Build history of the part. All positions in model axes, mm. A direction names the side the tool comes from. Round coordinates to 2 decimals unless told otherwise and drop trailing zeros. Loops run counter-clockwise (first coordinate to the right, second up) from the corner with the lowest first, then second, coordinate; pieces in that order, holes last.
from build123d import *

# Parameters (mm, degrees)
F0_W     = 6
F0_H     = 8.2
F0_W_2   = 17.4
F0_H_2   = 3
F1_DEPTH = 7.5


with BuildPart() as f1:
    # F0 (on Front) → F1 (new body, symmetric)
    with BuildSketch(Plane.XZ):
        Polygon((-49.911916, 14.810329), (-49.911916, 9.810329), (46.088084, 9.810329), (50.088084, 9.810329), (50.088084, 14.810329), (19.588084, 14.810329), (13.588084, 14.810329), (-43.911916, 14.810329), align=None)
        with Locations((16.588084, 18.910329)):
            Rectangle(F0_W, F0_H)
        with Locations((-46.911916, 18.910329)):
            Rectangle(F0_W, F0_H)
        Polygon((50.088084, 9.810329), (46.088084, 9.810329), (46.088084, -5.289671), (46.088084, -8.289671), (46.088084, -11.489671), (46.088084, -14.489671), (50.088084, -14.489671), align=None)
        with Locations((37.388084, -6.789671)):
            Rectangle(F0_W_2, F0_H_2)
        with Locations((37.388084, -12.989671)):
            Rectangle(F0_W_2, F0_H_2)
    extrude(amount=F1_DEPTH, both=True)


solid = f1.part
(1) Probe line 1 (Z direction, x = 32.5, y = 4); line 2 (X direction, y = -5.25, z = 20); line 3 (Z direction, x = 16, y = -7). List the from-to ranges inside material, lowest first.
Responses:
line 1: z = -14.49 to -11.49, -8.29 to -5.29, 9.81 to 14.81
line 2: x = -49.91 to -43.91, 13.59 to 19.59
line 3: z = 9.81 to 23.01
(2) Pull direction X, two halves, no side cores. Call faces 1 (the face through (28.688, 0, -13)), 2 (the face through (13.588, 0, 19)), 3 (the face through (-3, 0, 9.81)): +X half, -X half, draft (parallel to the pull), parting line (faces both ways), or undercut.
Responses:
face 1: -X half
face 2: undercut
face 3: draft
(3) Slice it at B-B on x = 31.5. List the corners of the cut face in (y, z).
Responses:
outline: (-7.5, -14.49) - (7.5, -14.49) - (7.5, -11.49) - (-7.5, -11.49) - close; (-7.5, -8.29) - (7.5, -8.29) - (7.5, -5.29) - (-7.5, -5.29) - close; (-7.5, 9.81) - (7.5, 9.81) - (7.5, 14.81) - (-7.5, 14.81) - close
(4) Slice it at C-C on y = 1.5. List the corners of the cut face in (x, z).
Responses:
outline: (-49.91, 9.81) - (46.09, 9.81) - (46.09, -5.29) - (28.69, -5.29) - (28.69, -8.29) - (46.09, -8.29) - (46.09, -11.49) - (28.69, -11.49) - (28.69, -14.49) - (50.09, -14.49) - (50.09, 14.81) - (19.59, 14.81) - (19.59, 23.01) - (13.59, 23.01) - (13.59, 14.81) - (-43.91, 14.81) - (-43.91, 23.01) - (-49.91, 23.01) - close
(5) Slice it at D-D on z = -3. List the corners of the cut face in (x, y), plus the area to 3 significant figures.
Responses:
outline: (46.09, -7.5) - (50.09, -7.5) - (50.09, 7.5) - (46.09, 7.5) - close
area: 60.0 mm2
(6) Pin check, flat tips, straight feed: P1, Ø1, axis at x = -38, y = -1.5, coming from the -Z side; P2, Ø1.5, axis at x = 29, z = -5, coming from the -Y side; P3, Ø1.5, axis at y = -3.5, z = -7, coming from the -X side; P4, Ø4.5, axis at x = 39, y = 2.5, coming from the +Z side. Stop position of each tip, or through.
Responses:
P1: stops at z = 9.81
P2: stops at y = -7.5
P3: stops at x = 28.69
P4: stops at z = 14.81
(7) Slice it at A-A on z = 18. List the corners of the cut face in (x, y), plus the area to 3 significant figures.
Responses:
outline: (-49.91, -7.5) - (-43.91, -7.5) - (-43.91, 7.5) - (-49.91, 7.5) - close; (13.59, -7.5) - (19.59, -7.5) - (19.59, 7.5) - (13.59, 7.5) - close
area: 180 mm2
(8) Which spindle directions (+Z, -Z, +X, -X, +Y, -Y) get a long thin tool onto all of the face, cutting with end or side? Do faces 4 (the face through (46.088, 0, 2)), 5 (the face through (-43.912, 0, 19)), 6 (the face through (35, 0, 14.81)), 7 (the face through (39, 0, -14.49)). Say none if no direction does.
Responses:
face 4: -X, +Y, -Y
face 5: +Z, +Y, -Y
face 6: +Z, +X, +Y, -Y
face 7: -Z, +X, -X, +Y, -Y
